from build123d import *

# Parameters (mm, degrees)
EXTRUDE_1_DEPTH     = 12.5
CUT_EXTRUDE_2_REACH = 29.819
SKETCH_6_R          = 6.25
EXTRUDE_2_DEPTH     = 4
SKETCH_7_R          = 1.5
EXTRUDE_3_DEPTH     = 3


with BuildPart() as part:
    # 草图1 → 凸台-拉伸1 (new body)
    with BuildSketch(Plane.XY):
        Polygon((-11.2, 11.4), (11.2, 11.4), (11.2, 7.7), (15.9, 7.7), (15.9, 4.7), (11.2, 4.7), (11.2, -11.4), (-11.2, -11.4), (-11.2, 4.7), (-15.9, 4.7), (-15.9, 7.7), (-11.2, 7.7), align=None)
    extrude(amount=EXTRUDE_1_DEPTH)

    # 草图5 → 切除-拉伸2 (cut, up to next)
    with BuildSketch(Plane(origin=(0, 7.7, 0), x_dir=(1, 0, 0), z_dir=(0, 1, 0)), mode=Mode.PRIVATE) as cut_extrude_2_sk1:
        with BuildLine():
            Line((-15.211065759, -6.75), (-15.9, -6.75))
            Line((-15.9, -6.75), (-15.9, -5.75))
            Line((-15.9, -5.75), (-15.211065759, -5.75))
            ThreePointArc((-15.211065759, -5.75), (-12.4, -6.25), (-15.211065759, -6.75))
        make_face()
    cut_extrude_2_tool1 = extrude(cut_extrude_2_sk1.sketch, amount=-CUT_EXTRUDE_2_REACH, mode=Mode.PRIVATE) & part.part
    cut_extrude_2 = cut_extrude_2_tool1.solids().sort_by_distance((-14.000898, 7.7, 6.25))[0]
    add(cut_extrude_2, mode=Mode.SUBTRACT)

    # 镜向2: 切除-拉伸2 across plane
    add(cut_extrude_2.mirror(Plane(origin=(0, 0, 0), x_dir=(0, 0, 1), z_dir=(1, 0, 0))), mode=Mode.SUBTRACT)

    # 草图6 → 凸台-拉伸2 (add)
    with BuildSketch(Plane(origin=(0, 11.4, 0), x_dir=(1, 0, 0), z_dir=(0, 1, 0))):
        with Locations((4.95, -6.25)):
            Circle(SKETCH_6_R)
    extrude(amount=EXTRUDE_2_DEPTH)

    # 草图7 → 凸台-拉伸3 (add)
    with BuildSketch(Plane(origin=(0, 15.4, 0), x_dir=(1, 0, 0), z_dir=(0, 1, 0))):
        with Locations(Location((4.95, -6.25, 0), (0, 0, 180))):
            Circle(SKETCH_7_R)
    extrude(amount=EXTRUDE_3_DEPTH)


solid = part.part
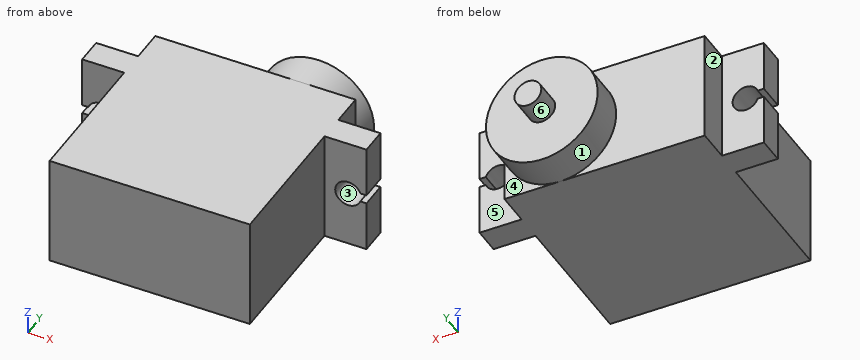
Build history of the part. All positions in model axes, mm. Face numbers are marked on the shaded views. A direction names the side the tool comes from. Coordinates: 2 decimals unless noted, no trailing zeros. Order: outer loops, then holes, each group sorted by start corner. A loop starts at its lowest first (then second) coordinate and runs counter-clockwise, first axis right, second up. Notation, with made-up numbers: M -39.75,73 L -16.75,73 A29 ccw -16.75,101 Z; hole C 77,59 d5. An arc over 180 degrees is marked long. One line per question, with ' | ' between items. Start each with the question number.
Q1. Saw through at D-D (x = 10). List the corners of the cut face in (y, z).
Q2. Two-plate mould, pull along Z, no slides. Class the marked faces 1, 2 and 3: +Z half, -Z half, draft (parallel to the pull), parting line (faces both ways), or undercut.
Q3. Saw through at A-A (x = -13.85). List the corners of the cut face in (y, z).
Q4. 3-axis set-ups, long thin cutter, end or side, ignore diameter. For the marked faces 4, 5 and 6: which of +Z, -Z, +X, -X, +Y, -Y reach the whole face in a straight line?
Q5. Probe L1, parallel to Z at x = 13.85, y = 6.5; L2, parallel to Y at x = 13, z = 8.75; L3, parallel to Y at x = -7, z = 1.75. List the from-to ranges inside material, lowest first. Write a range as from..to.
Q6. Flat gauge pins, fed straight in: pin 1 Ø5 at (x, y) = (7, 3.5) entering from -Z; pin 2 Ø1 at (y, z) = (-4, 2) entering from +X; pin 3 Ø5 at (x, z) = (-13.5, 7) entering from +Y; pin 4 Ø4 at (y, z) = (10.5, 9) entering from -X. Where does each tip first touch, or does it go through?
Q7. Saw through at C-C (z = 2). List the corners of the cut face in (x, y).
Q8. Saw through at B-B (z = 7.25). List the corners of the cut face in (x, y), then the cut area to 3 significant figures.
Check values:
1) outline: M -11.4,0 L 11.4,0 L 11.4,2.57 L 15.4,2.57 L 15.4,9.93 L 11.4,9.93 L 11.4,12.5 L -11.4,12.5 Z
2) face 1: parting line | face 2: draft | face 3: undercut
3) outline: M 4.7,0 L 7.7,0 L 7.7,4.8 L 4.7,4.8 Z; M 4.7,7.7 L 7.7,7.7 L 7.7,12.5 L 4.7,12.5 Z
4) face 4: -Z, +X, +Y | face 5: +Z, -Z, +X, +Y | face 6: +Y
5) L1: z = 0..4.8, 7.7..12.5 | L2: y = 4.7..7.7 | L3: y = -11.4..11.4
6) pin 1: stops at z = 0 | pin 2: stops at x = 11.2 | pin 3: stops at y = 11.4 | pin 4: stops at x = -11.2
7) outline: M -15.9,4.7 L -11.2,4.7 L -11.2,-11.4 L 11.2,-11.4 L 11.2,4.7 L 15.9,4.7 L 15.9,7.7 L 11.2,7.7 L 11.2,11.4 L 9.53,11.4 L 9.53,15.4 L 0.37,15.4 L 0.37,11.4 L -11.2,11.4 L -11.2,7.7 L -15.9,7.7 Z
8) outline: M -15.9,4.7 L -14.9,4.7 L -14.9,7.7 L -15.9,7.7 Z; M -12.8,4.7 L -11.2,4.7 L -11.2,-11.4 L 11.2,-11.4 L 11.2,4.7 L 12.8,4.7 L 12.8,7.7 L 11.2,7.7 L 11.2,11.4 L 11.12,11.4 L 11.12,15.4 L 6.07,15.4 L 6.07,18.4 L 3.83,18.4 L 3.83,15.4 L -1.22,15.4 L -1.22,11.4 L -11.2,11.4 L -11.2,7.7 L -12.8,7.7 Z; M 14.9,4.7 L 15.9,4.7 L 15.9,7.7 L 14.9,7.7 Z | area: 582 mm2
